Source: CAD feature listing. Evaluate the final solid. Frame: model axes, mm. Face numbers are marked on the shaded views. A direction names the side the tool comes from. Round coordinates to 2 decimals unless told otherwise and drop trailing zeros. Order: outer loops, then holes, each group sorted by start corner. A loop starts at its lowest first (then second) coordinate and runs counter-clockwise, first axis right, second up. Notation, with made-up numbers: (20.25, 15) - (62.25, 15) arc R14 ccw to (62.25, 20) - close; hole circle Ø11 at (33.5, 2). An arc over 180 degrees is marked (long way). Return JSON: item names as keys, results as strings. Group by question number.
1) Section B-B, the plane z = 0. Return loops of the section in (x, y).
2) Mould query, pull axis X, two halves, no side actions, for the marked faces 3, 4 and 5. Classes: pulls with the +X half, pulls with the -X half, needs draft (parallel to the pull), parting line crosses it, or undercut.
3) Section C-C, the plane y = 1.5. Return loops of the section in (x, z).
4) Access query for the marked faces 1 and 2. Directions: +Z, -Z, +X, -X, +Y, -Y. A direction counts if a zero-diameter tool reaches every point of the face in a straight line with its end or side. Return the directions, or none.
5) Ray query, line 1 (Z direction, x = 0, y = 2.1); line 2 (Z direction, x = -1, y = 1); line 3 (Y direction, x = -9.5, z = 18). Return the intervals inside material, ascending. Write a range as from..to.
6) Section D-D, the plane x = 20. Return loops of the section in (y, z), plus the area to 3 significant figures.
7) Contact query for flat-ended pins moving along their axis: P1, Ø2, axis at x = -10, y = 2, coming from the +Z side; P2, Ø6, axis at x = 0, z = 0, coming from the +Y side; P3, Ø6, axis at x = 0, z = 23.5, coming from the +Y side; P4, Ø10, axis at x = 13.5, y = 13, coming from the -Z side. Output: stop coordinate, or through.
8) Section A-A, the plane x = 0. Return loops of the section in (y, z).
```python
from build123d import *

# Parameters (mm, degrees)
SKETCH1_R           = 27.5
SKETCH1_R_2         = 5
SKETCH1_R_3         = 2.5
BOSS_EXTRUDE1_DEPTH = 3
SKETCH2_R           = 11.5
SKETCH2_R_2         = 5
BOSS_EXTRUDE2_DEPTH = 15


with BuildPart() as part:
    # Sketch1 → Boss-Extrude1 (new body)
    with BuildSketch(Plane(origin=(0, 0, 0), x_dir=(1, 0, 0), z_dir=(0, 1, 0))):
        Circle(SKETCH1_R)
        Circle(SKETCH1_R_2, mode=Mode.SUBTRACT)
        with Locations((0, 23.5)):
            Circle(SKETCH1_R_3, mode=Mode.SUBTRACT)
        with Locations((20.351596989, 11.75)):
            Circle(SKETCH1_R_3, mode=Mode.SUBTRACT)
        with Locations((20.351596989, -11.75)):
            Circle(SKETCH1_R_3, mode=Mode.SUBTRACT)
        with Locations((0, -23.5)):
            Circle(SKETCH1_R_3, mode=Mode.SUBTRACT)
        with Locations((-20.351596989, -11.75)):
            Circle(SKETCH1_R_3, mode=Mode.SUBTRACT)
        with Locations((-20.351596989, 11.75)):
            Circle(SKETCH1_R_3, mode=Mode.SUBTRACT)
    extrude(amount=BOSS_EXTRUDE1_DEPTH)

    # Sketch2 → Boss-Extrude2 (add)
    with BuildSketch(Plane(origin=(0, 3, 0), x_dir=(1, 0, 0), z_dir=(0, 1, 0))):
        Circle(SKETCH2_R)
        Circle(SKETCH2_R_2, mode=Mode.SUBTRACT)
    extrude(amount=BOSS_EXTRUDE2_DEPTH)


solid = part.part
```
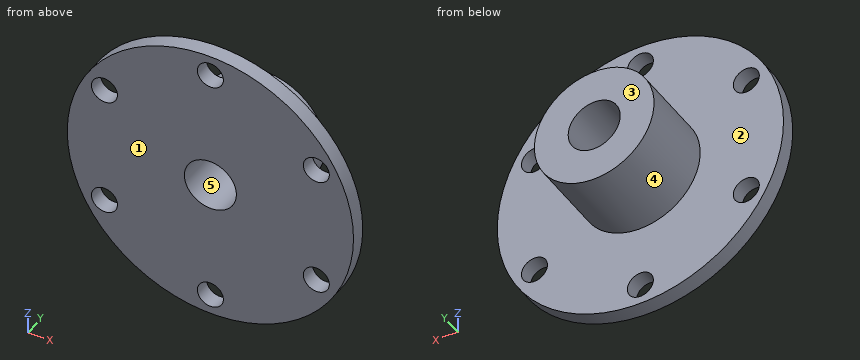
Geometry check:
{
 "1": {"outline": "(-27.5, 0) - (-5, 0) - (-5, 18) - (-11.5, 18) - (-11.5, 3) - (-27.5, 3) - close; (5, 0) - (27.5, 0) - (27.5, 3) - (11.5, 3) - (11.5, 18) - (5, 18) - close"},
 "2": {"face 3": "needs draft", "face 4": "parting line crosses it", "face 5": "undercut"},
 "3": {"outline": "circle Ø55 at (0, 0); hole circle Ø5 at (-20.35, -11.75); hole circle Ø5 at (-20.35, 11.75); hole circle Ø10 at (0, 0); hole circle Ø5 at (0, -23.5); hole circle Ø5 at (0, 23.5); hole circle Ø5 at (20.35, -11.75); hole circle Ø5 at (20.35, 11.75)"},
 "4": {"face 1": "+Z, -Z, +X, -X, -Y", "face 2": "+Y"},
 "5": {"line 1": "-27.5..-26, -21..-5, 5..21, 26..27.5", "line 2": "-27.48..-25.79, -21.21..-4.9, 4.9..21.21, 25.79..27.48", "line 3": "0..3"},
 "6": {"outline": "(0, -18.87) - (3, -18.87) - (3, -14.23) - (0, -14.23) - close; (0, -9.27) - (3, -9.27) - (3, 9.27) - (0, 9.27) - close; (0, 14.23) - (3, 14.23) - (3, 18.87) - (0, 18.87) - close", "area": "83.5 mm2"},
 "7": {"P1": "z = 25.99", "P2": "through", "P3": "y = 3", "P4": "z = -7.75"},
 "8": {"outline": "(0, -27.5) - (3, -27.5) - (3, -26) - (0, -26) - close; (0, -21) - (3, -21) - (3, -11.5) - (18, -11.5) - (18, -5) - (0, -5) - close; (0, 5) - (18, 5) - (18, 11.5) - (3, 11.5) - (3, 21) - (0, 21) - close; (0, 26) - (3, 26) - (3, 27.5) - (0, 27.5) - close"}
}
